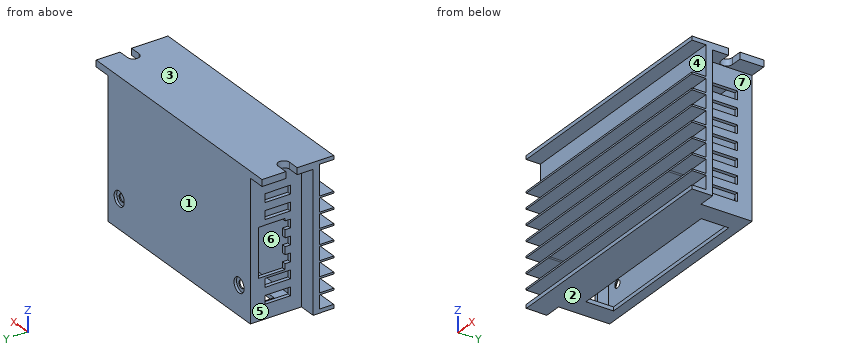
from build123d import *

# Parameters (mm, degrees)
SKETCH1_W                               = 95.3
SKETCH1_H                               = 56.8
BOSS_EXTRUDE1_DEPTH                     = 28.1
SKETCH2_W                               = 5.3
SKETCH2_H                               = 5.5
SKETCH2_W_2                             = 11.8
CUT_EXTRUDE2_DEPTH                      = 104.33566664
SKETCH3_W                               = 6.7
SKETCH3_H                               = 20
CUT_EXTRUDE4_DEPTH                      = 54.2
CUT_EXTRUDE5_DEPTH                      = 80.286647678
SKETCH5_W                               = 3.3
SKETCH5_H                               = 10
CUT_EXTRUDE6_DEPTH                      = 98.191203306
CUT_EXTRUDE8_REACH                      = 65.583
CUT_EXTRUDE8_START                      = -1.4
SKETCH6_W                               = 78.9
SKETCH6_H                               = 52.7
CUT_EXTRUDE9_REACH                      = 99.191
SKETCH7_W                               = 19
SKETCH7_H                               = 10.5
CUT_EXTRUDE10_REACH                     = 81.287
SKETCH8_W                               = 66.3
SKETCH8_H                               = 10.8
CBORE_FOR_M5_HEX_HEAD_BOLT1_D           = 3
CBORE_FOR_M5_HEX_HEAD_BOLT1_CBORE_D     = 5.8
CBORE_FOR_M5_HEX_HEAD_BOLT1_CBORE_DEPTH = 1


with BuildPart() as part:
    # Sketch1 → Boss-Extrude1 (new body)
    with BuildSketch(Plane(origin=(0, 0, 0), x_dir=(1, 0, 0), z_dir=(0, 1, 0))):
        Rectangle(SKETCH1_W, SKETCH1_H)
    extrude(amount=BOSS_EXTRUDE1_DEPTH)

    # Sketch2 → Cut-Extrude2 (cut, through all)
    with BuildSketch(Plane.ZY.offset(47.65)):
        with Locations((-24.25, 2.75)):
            Rectangle(SKETCH2_W, SKETCH2_H)
        with Locations((-18.25, 2.75)):
            Rectangle(SKETCH2_W, SKETCH2_H)
        with Locations((-12.25, 2.75)):
            Rectangle(SKETCH2_W, SKETCH2_H)
        with Locations((-6.25, 2.75)):
            Rectangle(SKETCH2_W, SKETCH2_H)
        with Locations((-0.25, 2.75)):
            Rectangle(SKETCH2_W, SKETCH2_H)
        with Locations((5.75, 2.75)):
            Rectangle(SKETCH2_W, SKETCH2_H)
        with Locations((11.75, 2.75)):
            Rectangle(SKETCH2_W, SKETCH2_H)
        with Locations((21, 2.75)):
            Rectangle(SKETCH2_W_2, SKETCH2_H)
    extrude(amount=-CUT_EXTRUDE2_DEPTH, mode=Mode.SUBTRACT)

    # Sketch3 → Cut-Extrude4 (cut)
    with BuildSketch(Plane(origin=(0, 0, -28.4), x_dir=(-1, 0, 0), z_dir=(0, 0, -1))):
        with Locations((-44.3, 18.1)):
            Rectangle(SKETCH3_W, SKETCH3_H)
        with Locations((44.3, 18.1)):
            Rectangle(SKETCH3_W, SKETCH3_H)
    extrude(amount=-CUT_EXTRUDE4_DEPTH, mode=Mode.SUBTRACT)

    # Sketch4 → Cut-Extrude5 (cut, through all)
    with BuildSketch(Plane.XY.offset(28.4)):
        with BuildLine():
            Line((43.3, 18.8), (52, 18.8))
            ThreePointArc((52, 18.8), (54.25, 16.55), (52, 14.3))
            Line((52, 14.3), (43.3, 14.3))
            ThreePointArc((43.3, 14.3), (41.05, 16.55), (43.3, 18.8))
        make_face()
    cut_extrude5 = extrude(amount=-CUT_EXTRUDE5_DEPTH, mode=Mode.SUBTRACT)

    # Mirror1: Cut-Extrude5 across plane
    add(cut_extrude5.mirror(Plane(origin=(0, 0, 0), x_dir=(0, 0, 1), z_dir=(1, 0, 0))), mode=Mode.SUBTRACT)

    # Sketch5 → Cut-Extrude6 (cut, through all)
    with BuildSketch(Plane(origin=(40.95, 0, 0), x_dir=(0, 0, -1), z_dir=(1, 0, 0))):
        with Locations((-16.55, 17.4)):
            Rectangle(SKETCH5_W, SKETCH5_H)
        with Locations((-10.25, 17.4)):
            Rectangle(SKETCH5_W, SKETCH5_H)
        with Locations((-3.95, 17.4)):
            Rectangle(SKETCH5_W, SKETCH5_H)
        with Locations((2.35, 17.4)):
            Rectangle(SKETCH5_W, SKETCH5_H)
        with Locations((8.65, 17.4)):
            Rectangle(SKETCH5_W, SKETCH5_H)
        with Locations((14.95, 17.4)):
            Rectangle(SKETCH5_W, SKETCH5_H)
        with Locations((21.25, 17.4)):
            Rectangle(SKETCH5_W, SKETCH5_H)
    extrude(amount=-CUT_EXTRUDE6_DEPTH, mode=Mode.SUBTRACT)

    # Cut-Extrude8: up to this face of the body (flat: up to its plane)
    cut_extrude8_end = Plane(part.part.faces().sort_by_distance((-44.3, 8.1, -1.3))[0])
    # Sketch6 → Cut-Extrude8 (cut, up to the picked face)
    with BuildSketch(Plane(origin=(0, 28.1, 0), x_dir=(1, 0, 0), z_dir=(0, 1, 0)).offset(CUT_EXTRUDE8_START), mode=Mode.PRIVATE) as cut_extrude8_sk1:
        with Locations((0, 0.55)):
            Rectangle(SKETCH6_W, SKETCH6_H)
    cut_extrude8_tool1 = split(extrude(cut_extrude8_sk1.sketch, amount=-CUT_EXTRUDE8_REACH, mode=Mode.PRIVATE), bisect_by=cut_extrude8_end, keep=Keep.BOTH, mode=Mode.PRIVATE)
    add(cut_extrude8_tool1.solids().sort_by(Axis((0, 26.7, -0.55), (0, -1, 0)))[0], mode=Mode.SUBTRACT)

    # Sketch7 → Cut-Extrude9 (cut, up to next)
    with BuildSketch(Plane.ZY.offset(40.95), mode=Mode.PRIVATE) as cut_extrude9_sk1:
        with Locations((-3, 19.75)):
            Rectangle(SKETCH7_W, SKETCH7_H)
    cut_extrude9_tool1 = extrude(cut_extrude9_sk1.sketch, amount=-CUT_EXTRUDE9_REACH, mode=Mode.PRIVATE) & part.part
    add(cut_extrude9_tool1.solids().sort_by_distance((-40.95, 19.75, -3))[0], mode=Mode.SUBTRACT)

    # Sketch8 → Cut-Extrude10 (cut, up to next)
    with BuildSketch(Plane(origin=(0, 0, -28.4), x_dir=(-1, 0, 0), z_dir=(0, 0, -1)), mode=Mode.PRIVATE) as cut_extrude10_sk1:
        with Locations((0, 18.9)):
            Rectangle(SKETCH8_W, SKETCH8_H)
    cut_extrude10_tool1 = extrude(cut_extrude10_sk1.sketch, amount=-CUT_EXTRUDE10_REACH, mode=Mode.PRIVATE) & part.part
    add(cut_extrude10_tool1.solids().sort_by_distance((0, 18.9, -28.4))[0], mode=Mode.SUBTRACT)

    # CBORE for M5 Hex Head Bolt1 (through all)
    with Locations(Plane(origin=(0, 28.1, 0), x_dir=(1, 0, 0), z_dir=(0, 1, 0))):
        with Locations((-34.45, 17)):
            cbore_for_m5_hex_head_bolt1 = CounterBoreHole(CBORE_FOR_M5_HEX_HEAD_BOLT1_D / 2, CBORE_FOR_M5_HEX_HEAD_BOLT1_CBORE_D / 2, CBORE_FOR_M5_HEX_HEAD_BOLT1_CBORE_DEPTH)

    # Mirror2: CBORE for M5 Hex Head Bolt1 across plane
    add(cbore_for_m5_hex_head_bolt1.mirror(Plane(origin=(0, 0, 0), x_dir=(0, 0, 1), z_dir=(1, 0, 0))), mode=Mode.SUBTRACT)


solid = part.part
Geometry check sheet. Reference: the model listing, model coordinates, mm. Face numbers are marked on the shaded views. A direction names the side the tool comes from. Coordinates: 2 decimals unless noted, no trailing zeros. Answer in a Markdown table with one row per item. Add a question column.
1) Set-up check for the marked faces 5, 6 and 7: record each of +Z, -Z, +X, -X, +Y, -Y from which the full face is reachable in a straight line by a thin tool's end or side.
2) Gauge pin test, flat ends, axial feed: P1, Ø1.2, axis at y = 18, z = -28, coming from the -X side; P2, Ø10, axis at y = 22, z = -5, coming from the -X side; P3, Ø5, axis at x = -34.45, z = -17, coming from the +Y side. Record the tip position at first contact, or that the pin passes through.
3) Release check for a two-part mould opening along Z. For the marked faces 1, 2, 3 and 4 record: +Z half, -Z half, draft (parallel to the pull), parting line (faces both ways), or undercut.
4) Cross-section at A-A, the plane y = 16.55. State how many separate pieces and enclosed holes the cut face has, then the cut area to 3 significant figures.
5) Material ranges on line 1 along X through (y, z) = (26.9, -17); line 2 along Y through (x, z) = (2.5, 5); line 3 along X through (y, z) = (27.3, -17), recorded low to high. Write a range as [from, to].
Check result:
| question | item | result |
|---|---|---|
| 1 | face 5 | -Z, -X, +Y |
| 1 | face 6 | none |
| 1 | face 7 | -Z, +X, +Y |
| 2 | P1 | stops at x = -40.95 |
| 2 | P2 | stops at x = -40.95 |
| 2 | P3 | stops at y = 27.1 |
| 3 | face 1 | draft |
| 3 | face 2 | -Z half |
| 3 | face 3 | +Z half |
| 3 | face 4 | undercut |
| 4 | separate pieces | 13 |
| 4 | enclosed holes | 0 |
| 4 | area | 312 mm² |
| 5 | line 1 | x = [-40.95, -35.95], [-32.95, 32.95], [35.95, 40.95] |
| 5 | line 2 | y = [5.5, 8.1], [26.7, 28.1] |
| 5 | line 3 | x = [-40.95, -37.35], [-31.55, 31.55], [37.35, 40.95] |
